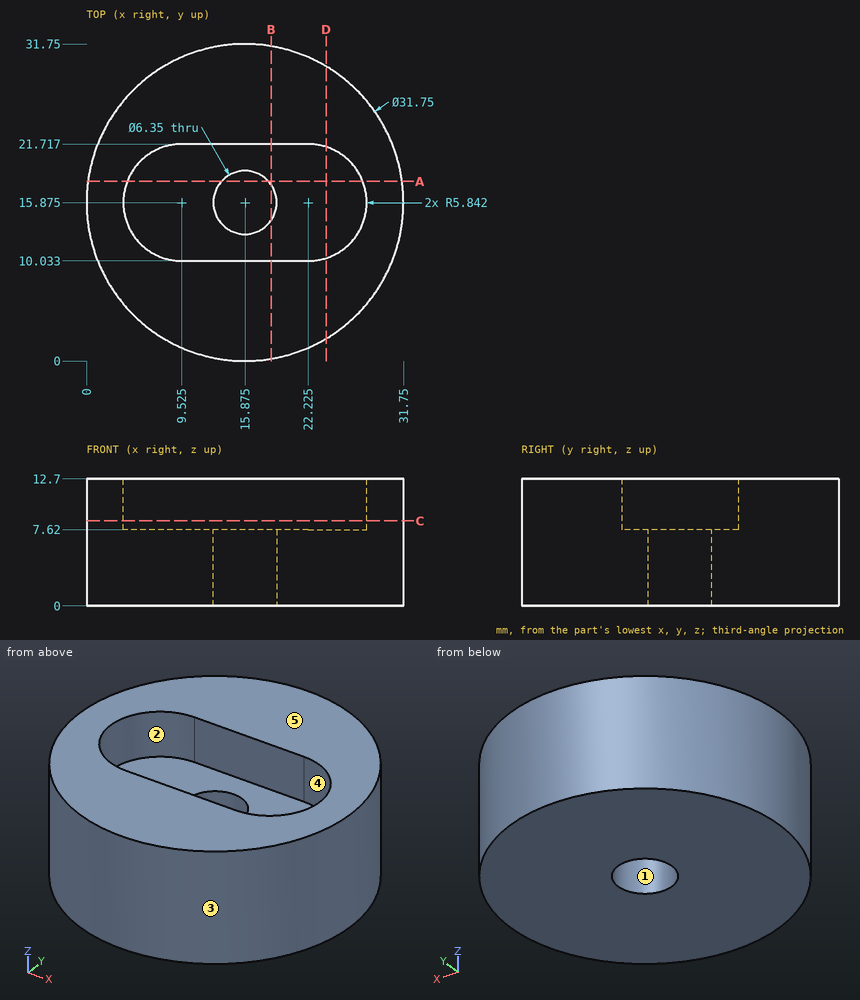
Geometry check sheet. Reference: drawing and pictorial views, mm from the part's lowest x, y, z. A direction names the side the tool comes from. Round coordinates to 2 decimals unless told otherwise and drop trailing zeros. Loops run counter-clockwise (first coordinate to the right, second up) from the corner with the lowest first, then second, coordinate; pieces in that order, holes last. Notation, with made-up numbers: M -30.5,23 L -5.5,23 A23 ccw -5.5,54 Z; hole C 5,-0.75 d3. An arc over 180 degrees is marked long. One line per item, written item: value.
(1) Release check for a two-part mould opening along Y. For the marked faces 3, 4 and 5 record: +Y half, -Y half, draft (parallel to the pull), parting line (faces both ways), or undercut.
Computed values:
face 3: parting line
face 4: undercut
face 5: draft
(2) Thickness scan on line 1 (Z direction, x = 13, y = 21); line 2 (X direction, y = 13, z = 4.25); line 3 (Y direction, x = 6, z = 7.75). Record the ranges inside material, lowest first.
Computed values:
line 1: z = 0 to 7.62
line 2: x = 0.26 to 14.53, 17.22 to 31.49
line 3: y = 3.45 to 11.22, 20.53 to 28.3
(3) Depth check by flat-ended pin: pin 1 Ø3 at (x, y) = (25, 16.5) entering from +Z; pin 2 Ø1 at (y, z) = (22, 5.5) entering from +X; pin 3 Ø1 at (y, z) = (23.5, 5) entering from -X. Enter the tip coordinate at first touch or a pass-through.
Computed values:
pin 1: stops at z = 7.62
pin 2: stops at x = 30.72
pin 3: stops at x = 1.69
(4) Sectioned sample at D-D, the plane x = 24. Record the cut outline in (y, z).
Computed values:
outline: M 2.24,0 L 29.51,0 L 29.51,12.7 L 21.44,12.7 L 21.44,7.62 L 10.31,7.62 L 10.31,12.7 L 2.24,12.7 Z
(5) Sectioned sample at B-B, the plane x = 18.5. Record the cut outline in (y, z), then the cut area to 3 significant figures.
Computed values:
outline: M 0.22,0 L 14.09,0 L 14.09,7.62 L 10.03,7.62 L 10.03,12.7 L 0.22,12.7 Z; M 17.66,0 L 31.53,0 L 31.53,12.7 L 21.72,12.7 L 21.72,7.62 L 17.66,7.62 Z
area: 311 mm^2
(6) Access from +Z, -Z, +X, -X, +Y, -Y to the whole of each face (thin tool, end or side, straight path). Record for the marked faces 1 and 2.
Computed values:
face 1: +Z, -Z
face 2: +Z
(7) Sectioned sample at A-A, the plane y = 18. Record the cut outline in (x, z).
Computed values:
outline: M 0.14,0 L 13.52,0 L 13.52,7.62 L 4.08,7.62 L 4.08,12.7 L 0.14,12.7 Z; M 18.23,0 L 31.61,0 L 31.61,12.7 L 27.67,12.7 L 27.67,7.62 L 18.23,7.62 Z
(8) Sectioned sample at C-C, the plane z = 8.5. Record the cut outline in (x, y) (3 decimals).
Computed values:
outline: C 15.875,15.875 d31.75; hole M 9.525,10.033 L 22.225,10.033 A5.842 ccw 22.225,21.717 L 9.525,21.717 A5.842 ccw Z
